from build123d import *

# Parameters (mm, degrees)
SKETCH2_W          = 38.1
SKETCH2_H          = 19.05
CUT_EXTRUDE1_DEPTH = 5.08
FILLET1_R          = 4.7625


with BuildPart() as part:
    # Sketch1 → Revolve1 (revolve)
    with BuildSketch(Plane.XY):
        Polygon((0, 0), (25.4, 0), (25.4, 19.05), (30.1625, 19.05), (30.1625, 44.45), (33.3375, 44.45), (33.3375, 4.7625), (30.1625, 4.7625), (30.1625, -7.9375), (0, -7.9375), align=None)
    revolve(axis=Axis((0, 0, 0), (0, -1, 0)))

    # Sketch2 → Cut-Extrude1 (cut)
    with BuildSketch(Plane(origin=(0, 0, 0), x_dir=(1, 0, 0), z_dir=(0, 1, 0))):
        Rectangle(SKETCH2_W, SKETCH2_H)
    extrude(amount=-CUT_EXTRUDE1_DEPTH, mode=Mode.SUBTRACT)

    # Fillet1
    fillet1_edges = [part.edges().sort_by_distance(p)[0] for p in [
        (19.05, -2.54, -9.525),
        (19.05, -2.54, 9.525),
        (-19.05, -2.54, 9.525),
        (-19.05, -2.54, -9.525),
    ]]
    fillet(fillet1_edges, radius=FILLET1_R)


solid = part.part
The listing builds one solid part. Answer for the finished solid, in the listing's coordinates (mm). A direction names the side the tool comes from. Coordinates: 2 decimals unless noted, no trailing zeros. Write each loop counter-clockwise with the first axis right and the second up, starting at its lowest first coordinate (ties: lowest second). Pieces come first, ordered by that corner, then holes. Notation, with made-up numbers: M 16.5,-36.75 L 41.5,-36.75 A25 ccw 41.5,-23.75 Z; hole C -23,20 d4. An arc over 180 degrees is marked long. Write each question's results on one line, items separated by ' | '.
Item 1: The part is cut by section C-C on z = 2.5. Determine the outline of the cut face in (x, y).
Answer below:
outline: M -33.24,4.76 L -30.06,4.76 L -30.06,-7.94 L 30.06,-7.94 L 30.06,4.76 L 33.24,4.76 L 33.24,44.45 L 30.06,44.45 L 30.06,19.05 L 25.28,19.05 L 25.28,0 L 19.05,0 L 19.05,-5.08 L -19.05,-5.08 L -19.05,0 L -25.28,0 L -25.28,19.05 L -30.06,19.05 L -30.06,44.45 L -33.24,44.45 Z
Item 2: Consider probe 1 along Z at (x, y) = (0, 31); probe 2 along Z at (x, y) = (0, 6); probe 3 along Y at (x, z) = (3.5, -2.5). Determine where each line is inside the solid, lowest interval first. Write a range as [from, to].
Answer below:
probe 1: [-33.34, -30.16], [30.16, 33.34] | probe 2: [-33.34, -25.4], [25.4, 33.34] | probe 3: [-7.94, -5.08]
Item 3: The part is cut by section D-D on y = 34.5. Determine the outline of the cut face in (x, z) (1 decimal).
Answer below:
outline: C 0,0 d66.7; hole C 0,0 d60.3
Item 4: Given P1, Ø5, axis at x = -16, y = 26.5, coming from the -Z side; P2, Ø1.5, axis at x = -13.5, z = 17, coming from the +Y side; P3, Ø5.5, axis at y = -1.5, z = 1, coming from the +X side, each flat-ended and moving along its own axis, determine where each tip first touches the part or whether it passes through.
Answer below:
P1: z = -30.48 | P2: y = 0 | P3: x = 30.16
Item 5: For a pull along Z with two mould halves and no side action, classify faces 4 (the face through (19.05, -3, 0)), 5 (the face through (7.6, 44.45, -29.5)), 6 (the face through (31.8, 24.33, 10.01)) as released by +Z, released by -Z, zero draft, split by the parting line, or undercut.
Answer below:
face 4: undercut | face 5: zero draft | face 6: split by the parting line
Item 6: Which of the six approach directions +Z, -Z, +X, -X, +Y, -Y give full straight-line access (tool end or side, diameter ignored) to faces 1 (the face through (0, -7.938, 0)), 2 (the face through (-7.6, 4.762, -29.5)), 3 (the face through (0, -5.08, 0))?
Answer below:
face 1: +Z, -Z, +X, -X, -Y | face 2: -Y | face 3: +Y
